Build history of the part. All positions in model axes, mm. Give positions to 0.01 mm unless a question says otherwise; leave off trailing zeros. Loops run counter-clockwise (first coordinate to the right, second up) from the corner with the lowest first, then second, coordinate; pieces in that order, holes last. Notation, with made-up numbers: M -18,8 L 16,8 A15 cw 16,14 Z; hole C -15.5,29 d7. An arc over 180 degrees is marked long. Answer as a JSON object with one key per item and string values. Group by question number.
1. Slice it at B-B (y = -7). List the corners of the cut face in (x, z), then the cut area to 3 significant figures.
2. Mould opens along X. For faces 1 (the face through (0.314, -8.416, -0.74)), 2 (the face through (1.5, 0.07, -0.74)), 3 (the face through (-0.867, -3.905, 1.232)), 4 (the face through (-5, 0, 0)) say: released by +X, released by -X, zero draft, split by the parting line, or undercut.
3. Drill centre lines: line 1 along Y through (x, z) = (0, -0.4); line 2 along Z through (x, y) = (-3, -5); line 3 along Y through (x, z) = (7, -0.5). Where is each one in solid material? Low to high. Write a range as [from, to].
4. Slice it at C-C (z = -0.3). List the corners of the cut face in (x, y), then the cut area to 3 significant figures.
5. Drop flat-ended pins along their axis: pin 1 Ø1.5 at (x, z) = (3, -0.5) entering from -Y; pin 2 Ø4 at (x, y) = (0, 0) entering from +Z; pin 3 Ø1.5 at (y, z) = (-4.5, -0.5) entering from -X. Give the stop position or say it passes through.
6. Slice it at D-D (y = -4.5). List the corners of the cut face in (x, z).
7. Slice it at A-A (x = 7.25). List the corners of the cut face in (y, z), then the cut area to 3 significant figures.
from build123d import *

# Parameters (mm, degrees)
SKETCH_1_R      = 4
EXTRUDE_1_DEPTH = 2.5
SKETCH_2_R      = 11.75
SKETCH_2_R_2    = 1.45
SKETCH_2_R_3    = 1.5
EXTRUDE_2_DEPTH = 1.5


with BuildPart() as part:
    # 草图1 → 凸台-拉伸1 (new body)
    with BuildSketch(Plane.XY):
        Circle(SKETCH_1_R)
        Polygon((0, 2.25), (0.358703838, 2.839433251), (0.559552246, 2.179312113), (1.053572832, 2.661021217), (1.083945767, 1.97169003), (1.68224197, 2.315407433), (1.540230988, 1.640179412), (2.205209658, 1.824308085), (1.899737832, 1.205610289), (2.589615914, 1.218580751), (2.139877162, 0.695288237), (2.811307077, 0.536285507), (2.245560139, 0.141278669), (2.856353478, -0.179706529), (2.210146314, -0.421607958), (2.721924685, -0.884406942), (2.035860868, -0.958003406), (2.416467353, -1.533536814), (1.733654796, -1.434203977), (1.95917449, -2.086308928), (1.322516818, -1.820288237), (1.378779489, -2.50799058), (0.828280244, -2.091997093), (0.711750702, -2.772085959), (0.281999776, -2.232258078), (0, -2.862000983), (-0.281999776, -2.232258078), (-0.711750702, -2.772085959), (-0.828280244, -2.091997093), (-1.378779489, -2.50799058), (-1.322516818, -1.820288237), (-1.95917449, -2.086308928), (-1.733654796, -1.434203977), (-2.416467353, -1.533536814), (-2.035860868, -0.958003406), (-2.721924685, -0.884406942), (-2.210146314, -0.421607958), (-2.856353478, -0.179706529), (-2.245560139, 0.141278669), (-2.811307077, 0.536285507), (-2.139877162, 0.695288237), (-2.589615914, 1.218580751), (-1.899737832, 1.205610289), (-2.205209658, 1.824308085), (-1.540230988, 1.640179412), (-1.68224197, 2.315407433), (-1.083945767, 1.97169003), (-1.053572832, 2.661021217), (-0.559552246, 2.179312113), (-0.358703838, 2.839433251), align=None, mode=Mode.SUBTRACT)
    extrude(amount=EXTRUDE_1_DEPTH)

    # 草图2 → 凸台-拉伸2 (add)
    with BuildSketch(Plane(origin=(0, 0, 0), x_dir=(-1, 0, 0), z_dir=(0, 0, -1))):
        Circle(SKETCH_2_R)
        with Locations((-7, 0)):
            Circle(SKETCH_2_R_2, mode=Mode.SUBTRACT)
        with Locations((0, 7)):
            Circle(SKETCH_2_R_2, mode=Mode.SUBTRACT)
        with Locations((7, 0)):
            Circle(SKETCH_2_R_2, mode=Mode.SUBTRACT)
        with Locations((0, -7)):
            Circle(SKETCH_2_R_2, mode=Mode.SUBTRACT)
        Circle(SKETCH_2_R_3, mode=Mode.SUBTRACT)
    extrude(amount=EXTRUDE_2_DEPTH)


solid = part.part
Established:
{
 "1": {"outline": "M -9.44,-1.5 L -1.45,-1.5 L -1.45,0 L -9.44,0 Z; M 1.45,-1.5 L 9.44,-1.5 L 9.44,0 L 1.45,0 Z", "area": "24.0 mm^2"},
 "2": {"face 1": "undercut", "face 2": "undercut", "face 3": "split by the parting line", "face 4": "zero draft"},
 "3": {"line 1": "y = [-11.75, -8.45], [-5.55, -1.5], [1.5, 5.55], [8.45, 11.75]", "line 2": "z = [-1.5, 0]", "line 3": "y = [-9.44, -1.45], [1.45, 9.44]"},
 "4": {"outline": "C 0,0 d23.5; hole C -7,0 d2.9; hole C 0,0 d3; hole C 0,-7 d2.9; hole C 0,7 d2.9; hole C 7,0 d2.9", "area": "400 mm^2"},
 "5": {"pin 1": "stops at y = -11.53", "pin 2": "stops at z = 0", "pin 3": "stops at x = -11.14"},
 "6": {"outline": "M -10.85,-1.5 L 10.85,-1.5 L 10.85,0 L -10.85,0 Z"},
 "7": {"outline": "M -9.25,-1.5 L -1.43,-1.5 L -1.43,0 L -9.25,0 Z; M 1.43,-1.5 L 9.25,-1.5 L 9.25,0 L 1.43,0 Z", "area": "23.5 mm^2"}
}
